Geometry: final body of the model. Coordinates: model frame, mm. A direction names the side the tool comes from. Give positions to 0.01 mm unless a question says otherwise; leave off trailing zeros. Write each loop counter-clockwise with the first axis right and the second up, starting at its lowest first coordinate (ties: lowest second). Pieces come first, ordered by that corner, then holes.
Q1. Line query: L1, parallel to Y at x = 5.25, z = 22; L2, parallel to X at y = -8.75, z = 38; L3, parallel to Z at x = -1, y = -2.75. Output: solid intervals per line, ascending.
Q2. Cut plane B-B on y = -5.5. Return the cut outline in (x, z), plus the area to 3 significant figures.
Q3. Cut plane C-C on z = 42.5. Return the cut outline in (x, y), plus the area to 3 significant figures.
Q4. Reachability of faces 1 (the face through (-5, 0, 18)), 2 (the face through (0, 1.14, 23)), 3 (the face through (0, -11.14, 23)), 4 (the face through (3.728, -4.93, 34.375)), 5 (the face through (5, 0, 18)) from +Z, -Z, +X, -X, +Y, -Y: full face, straight path, thin tool, end or side. Return the list, or none.
Q5. Draft query along X for faces 6 (the face through (0, -10, 28)), 7 (the face through (5, -5, 40)), 8 (the face through (6.35, -10.4, 32.2)), 9 (the face through (-4.951, -4.93, 34.014)). Return one class per face: pulls with the +X half, pulls with the -X half, needs draft (parallel to the pull), parting line crosses it, or undercut.
Q6. Cut plane D-D on z = 32.5. Return the cut outline in (x, y), plus the area to 3 significant figures.
Q7. Cut plane A-A on x = 0. Return the cut outline in (y, z).
Q8. Pin query (flat end, axial travel): pin 1 (2.5 mm diameter, centred on x = 0.5, y = -6, fed in from +Z). Return the tip coordinate at first contact, or that it passes through.
```python
from build123d import *

# Parameters (mm, degrees)
F1_DEPTH = 10
F2_W     = 12.7
F2_H     = 45
F3_DEPTH = 1.14
F4_W     = 12.7
F4_H     = 45
F5_DEPTH = 1.14


with BuildPart() as f1:
    # F0 (on Front) → F1 (new body)
    with BuildSketch(Plane.XZ):
        Polygon((-5, 45), (-6.35, 45), (-6.35, 35), (-3.511587, 33), (-3.44, 0), (0, 0), (0, 1.69), (-2.35, 1.69), (-2.418905, 33.453385), (-5, 35.272074), align=None)
        Polygon((0, 1.69), (0, 0), (3.44, 0), (3.511587, 33), (6.35, 35), (6.35, 45), (5, 45), (5, 35.272074), (2.418905, 33.453385), (2.35, 1.69), align=None)
    extrude(amount=F1_DEPTH)

    # F2 (on Front) → F3 (join)
    with BuildSketch(Plane.XZ):
        with Locations((0, 22.5)):
            Rectangle(F2_W, F2_H)
    extrude(amount=-F3_DEPTH)

    # F4 (on face) → F5 (join)
    with BuildSketch(Plane.XZ.offset(10)):
        with Locations((0, 22.5)):
            Rectangle(F4_W, F4_H)
    extrude(amount=F5_DEPTH)


solid = f1.part
```
Data:
1. L1: y = -11.14 to -10, 0 to 1.14
1. L2: x = -6.35 to -5, 5 to 6.35
1. L3: z = 0 to 1.69
2. outline: (-6.35, 35) - (-3.51, 33) - (-3.44, 0) - (3.44, 0) - (3.51, 33) - (6.35, 35) - (6.35, 45) - (5, 45) - (5, 35.27) - (2.42, 33.45) - (2.35, 1.69) - (-2.35, 1.69) - (-2.42, 33.45) - (-5, 35.27) - (-5, 45) - (-6.35, 45) - close
2. area: 114 mm2
3. outline: (-6.35, -11.14) - (6.35, -11.14) - (6.35, 1.14) - (-6.35, 1.14) - close; hole (-5, -10) - (5, -10) - (5, 0) - (-5, 0) - close
3. area: 56.0 mm2
4. face 1: -Z, -X
4. face 2: +Z, -Z, +X, -X, +Y
4. face 3: +Z, -Z, +X, -X, -Y
4. face 4: +Z
4. face 5: -Z, +X
5. face 6: undercut
5. face 7: undercut
5. face 8: pulls with the +X half
5. face 9: pulls with the -X half
6. outline: (-6.35, -11.14) - (6.35, -11.14) - (6.35, -10) - (3.51, -10) - (3.51, 0) - (6.35, 0) - (6.35, 1.14) - (-6.35, 1.14) - (-6.35, 0) - (-3.51, 0) - (-3.51, -10) - (-6.35, -10) - close; hole (-2.42, -10) - (2.42, -10) - (2.42, 0) - (-2.42, 0) - close
6. area: 50.8 mm2
7. outline: (-11.14, 0) - (1.14, 0) - (1.14, 45) - (0, 45) - (0, 1.69) - (-10, 1.69) - (-10, 45) - (-11.14, 45) - close
8. pin 1: stops at z = 1.69
